Autodesk Inventor part; units mm, degrees
ref_plane "Start plane" through (0, 0, 0) normal (0, 0, 1) x (1, 0, 0)
ref_plane "End plane" through (0, 0, 330) normal (0, 0, 1) x (1, 0, 0)
ref_plane "Work Plane4" through (39.5, -55, 0) normal (0, 0, -1) x (-1, 0, 0)
ref_plane "Start plane" through (0, 0, 0) normal (0, 0, 1) x (1, 0, 0)
ref_plane "End plane" through (0, 0, 330) normal (0, 0, 1) x (1, 0, 0)
sketch "Sketch" plane through (0, 0, 0) normal (0, 0, 1) x (1, 0, 0)
  line L0 (-7.5, -7.75) -> (-7.5, 7.75)
  line L1 (-5.25, 10) -> (5.25, 10)
  line L2 (7.5, 7.75) -> (7.5, -7.75)
  line L3 (5.25, -10) -> (-5.25, -10)
  arc A0 (-7.5, -7.75) -> (-5.25, -10) centre (-5.25, -7.75) ccw
  arc A1 (-5.25, 10) -> (-7.5, 7.75) centre (-5.25, 7.75) ccw
  arc A2 (7.5, 7.75) -> (5.25, 10) centre (5.25, 7.75) ccw
  arc A3 (5.25, -10) -> (7.5, -7.75) centre (5.25, -7.75) ccw
  arc A4 (-5.25, 8.5) -> (-6, 7.75) centre (-5.25, 7.75) ccw
  line L4 (-5.25, 8.5) -> (5.25, 8.5)
  arc A5 (6, 7.75) -> (5.25, 8.5) centre (5.25, 7.75) ccw
  line L5 (6, 7.75) -> (6, -7.75)
  arc A6 (5.25, -8.5) -> (6, -7.75) centre (5.25, -7.75) ccw
  line L6 (5.25, -8.5) -> (-5.25, -8.5)
  arc A7 (-6, -7.75) -> (-5.25, -8.5) centre (-5.25, -7.75) ccw
  line L7 (-6, -7.75) -> (-6, 7.75)
  line L8 (0, 14.6524) -> (0, -14.6524) construction
  line L9 (-11.5592, 0) -> (13.5932, 0) construction
  dimension "d7" = 2.25
  dimension "d10" = 20
  dimension "d11" = 15
  dimension "d12" = 1.5
  dimension "d15" = 10
  dimension "d16" = 7.5
extrude "Body" add sketch "Sketch" along normal up to surface (330 mm away) from surface at 0
sketch "Sketch3" plane through (0, 0, 0) normal (0, 0, 1) x (1, 0, 0)
  line L0 (0, 0) -> (10, 0)
ref_plane "Work Plane3" through (0, 0, 0) normal (0, -1, 0) x (1, 0, 0)
sketch "Sketch4" plane through (0, 0, 0) normal (0, -1, 0) x (1, 0, 0)
  line L0 (-2, 0) -> (12, 0)
  line L1 (-2, 330) -> (12, 330)
  dimension "d18" = 330
ref_plane "Work Plane4" through (39.5, -55, 0) normal (0, 0, -1) x (-1, 0, 0)
split "Split1" plane through (39.5, -55, 0) removes the side toward (0, 0, -1)
ref_plane "Work Plane5" through (-4.5, -55, 330) normal (0, 0, 1) x (1, 0, 0)
split "Split2" plane through (-4.5, -55, 330) removes the side toward (0, 0, 1)
equation "\"d7\" = G_IR"
equation "\"d10\" = G_H"
equation "\"d11\" = G_W"
equation "\"d12\" = G_T"
equation "\"d15\" = 0.5 * d10"
equation "\"d16\" = 0.5 * d11"
equation "\"d3\" = G_L"
equation "\"G_W\" = 15"
equation "\"G_H\" = 20"
equation "\"G_T\" = 1.5"
equation "\"G_IR\" = 2.25"
equation "\"G_L\" = d18"
equation "\"G_OFFSET_START\" = 0"
equation "\"G_OFFSET_END\" = -40"
equation "\"d14\" = G_OFFSET_END + B_L"
equation "\"B_L\" = 370"
properties part number "UNI EN 10305-5 - 20 x 15 x 1,5  - 330" material "Steel, Mild"
Part model, mm, in its own coordinate system. A direction names the side the tool comes from. Round coordinates to 2 decimals unless told otherwise and drop trailing zeros. Loops run counter-clockwise (first coordinate to the right, second up) from the corner with the lowest first, then second, coordinate; pieces in that order, holes last.
Item 1: Cut at B-B, the plane z = 196. Give the cut face in (x, y), then the cut area to 3 significant figures.
Item 2: Cut at A-A, the plane x = 2.5. Give the cut face in (y, z), then the cut area to 3 significant figures.
Item 3: 3-axis set-ups, long thin cutter, end or side, ignore diameter. For faces 1 (the face through (0, -8.5, 163)), 2 (the face through (7.5, 0, 163)): which of +Z, -Z, +X, -X, +Y, -Y reach the whole face in a straight line?
Item 4: Drill centre lines: line 1 (X direction, y = 7, z = 315.5); line 2 (Y direction, x = 1.75, z = 257); line 3 (Y direction, x = 5.75, z = 261.5). Where is each one in solid material? Low to high.
Item 5: Drop a flat-ended pin along its axis: P1, Ø4, axis at x = -5.5, z = 143.5, coming from the +Y side. Give the stop position or say it passes through.
Item 6: Mould opens along Y. For faces 3 (the face through (0, -10, 163)), 4 (the face through (-7, 0, 330)), 5 (the face through (6, 0, 163)), 6 (the face through (0, 10, 163)) say: +Y half, -Y half, draft (parallel to the pull), parting line (faces both ways), or undercut.
Item 7: Cut at C-C, the plane y = -4.5. Give the cut face in (x, z).
A:
1. outline: (-7.5, -7.75) arc R2.25 ccw to (-5.25, -10) - (5.25, -10) arc R2.25 ccw to (7.5, -7.75) - (7.5, 7.75) arc R2.25 ccw to (5.25, 10) - (-5.25, 10) arc R2.25 ccw to (-7.5, 7.75) - close; hole (-6, -7.75) arc R0.75 ccw to (-5.25, -8.5) - (5.25, -8.5) arc R0.75 ccw to (6, -7.75) - (6, 7.75) arc R0.75 ccw to (5.25, 8.5) - (-5.25, 8.5) arc R0.75 ccw to (-6, 7.75) - close
1. area: 92.1 mm2
2. outline: (-10, 0) - (-8.5, 0) - (-8.5, 330) - (-10, 330) - close; (8.5, 0) - (10, 0) - (10, 330) - (8.5, 330) - close
2. area: 990 mm2
3. face 1: +Z, -Z
3. face 2: +Z, -Z, +X, +Y, -Y
4. line 1: x = -7.5 to -6, 6 to 7.5
4. line 2: y = -10 to -8.5, 8.5 to 10
4. line 3: y = -9.94 to -8.31, 8.31 to 9.94
5. P1: stops at y = 10
6. face 3: -Y half
6. face 4: draft
6. face 5: undercut
6. face 6: +Y half
7. outline: (-7.5, 0) - (-6, 0) - (-6, 330) - (-7.5, 330) - close; (6, 0) - (7.5, 0) - (7.5, 330) - (6, 330) - close
